from build123d import *

# Parameters (mm, degrees)
F1_DEPTH = 35
F3_DEPTH = 30.001


with BuildPart() as f1:
    # F0 (on Front) → F1 (new body)
    with BuildSketch(Plane.XZ):
        Polygon((0, 30), (0, 0), (12, 0), (12, 18), (78, 18), (78, 0), (90, 0), (90, 30), align=None)
    extrude(amount=F1_DEPTH)

    # F2 (on face) → F3 (cut, through all)
    with BuildSketch(Plane.XY.offset(30)):
        with BuildLine():
            Line((37, 0), (37, -15))
            ThreePointArc((37, -15), (45, -23), (53, -15))
            Line((53, -15), (53, 0))
            Line((53, 0), (37, 0))
        make_face()
    extrude(amount=-F3_DEPTH, mode=Mode.SUBTRACT)


solid = f1.part
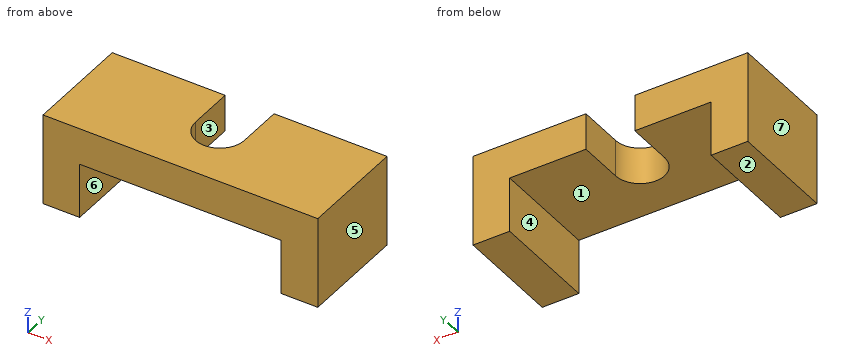
Design review of the part built by this model. Coordinates are the model's own, in mm. Face numbers are marked on the shaded views. A direction names the side the tool comes from. Round coordinates to 2 decimals unless told otherwise and drop trailing zeros. Write each loop counter-clockwise with the first axis right and the second up, starting at its lowest first coordinate (ties: lowest second). Pieces come first, ordered by that corner, then holes. Notation, with made-up numbers: M 75,48.25 L 84,48.25 A21 cw 84,84.25 Z; hole C 71,57 d8. An arc over 180 degrees is marked long. One line per item, written item: value. Start each with the question number.
1. Clearance check with a flat-ended pin moving along its axis: P1, Ø8, axis at x = 47.5, y = -23.5, coming from the -Z side. State where the tip first meets the part, or that it passes through.
2. To check wall thickness, follow probe 1 along X at (y, z) = (-11.5, 23.25); probe 2 along X at (y, z) = (-22, 3.5); probe 3 along Z at (x, y) = (42.5, -25.5). State the ranges of each line that lie inside material, in increasing order. Write a range as from..to.
3. Draft analysis for pull direction X (two halves, no side actions). For the marked faces 4, 5, 6 and 7, state which applies: pulls with the +X half, pulls with the -X half, needs draft (parallel to the pull), parting line crosses it, or undercut.
4. Take a section at B-B on z = 11.75. State the section outline as (x, y) points, then the cut area to 3 significant figures.
5. Take a section at C-C on z = 26.25. State the section outline as (x, y) points, then the cut area to 3 significant figures.
6. Take a section at D-D on y = -30.5. State the section outline as (x, z) points, then the cut area to 3 significant figures.
7. For the marked faces 1, 2 and 3, list the 3-axis set-ups (+Z, -Z, +X, -X, +Y, -Y) from which the entire face can be reached by the end or side of a thin tool; tool diameter is ignored.
8. Take a section at A-A on y = -3.5. State the section outline as (x, z) points.
Computed:
1. P1: stops at z = 18
2. probe 1: x = 0..37, 53..90
2. probe 2: x = 0..12, 78..90
2. probe 3: z = 18..30
3. face 4: undercut
3. face 5: pulls with the +X half
3. face 6: undercut
3. face 7: pulls with the -X half
4. outline: M 0,-35 L 12,-35 L 12,0 L 0,0 Z; M 78,-35 L 90,-35 L 90,0 L 78,0 Z
4. area: 840 mm²
5. outline: M 0,-35 L 90,-35 L 90,0 L 53,0 L 53,-15 A8 cw 37,-15 L 37,0 L 0,0 Z
5. area: 2,810 mm²
6. outline: M 0,0 L 12,0 L 12,18 L 78,18 L 78,0 L 90,0 L 90,30 L 0,30 Z
6. area: 1,510 mm²
7. face 1: -Z, +Y, -Y
7. face 2: -Z, +X, -X, +Y, -Y
7. face 3: +Z, -Z, +Y
8. outline: M 0,0 L 12,0 L 12,18 L 37,18 L 37,30 L 0,30 Z; M 53,18 L 78,18 L 78,0 L 90,0 L 90,30 L 53,30 Z
